Geometry: see drawing. Coordinates: mm, zero at the bounding-box minimum. A direction names the side the tool comes from. Coordinates: 2 decimals unless noted, no trailing zeros. Order: outer loops, then holes, each group sorted by start corner. A loop starts at its lowest first (then second) coordinate and runs counter-clockwise, first axis right, second up. Notation, with made-up numbers: (21, 51) -> (41, 51) arc R20 ccw to (41, 67) -> close; hole circle Ø10 at (75.25, -8). An arc over 180 degrees is marked (long way). Write each question's results on one line, items separated by ' | '.
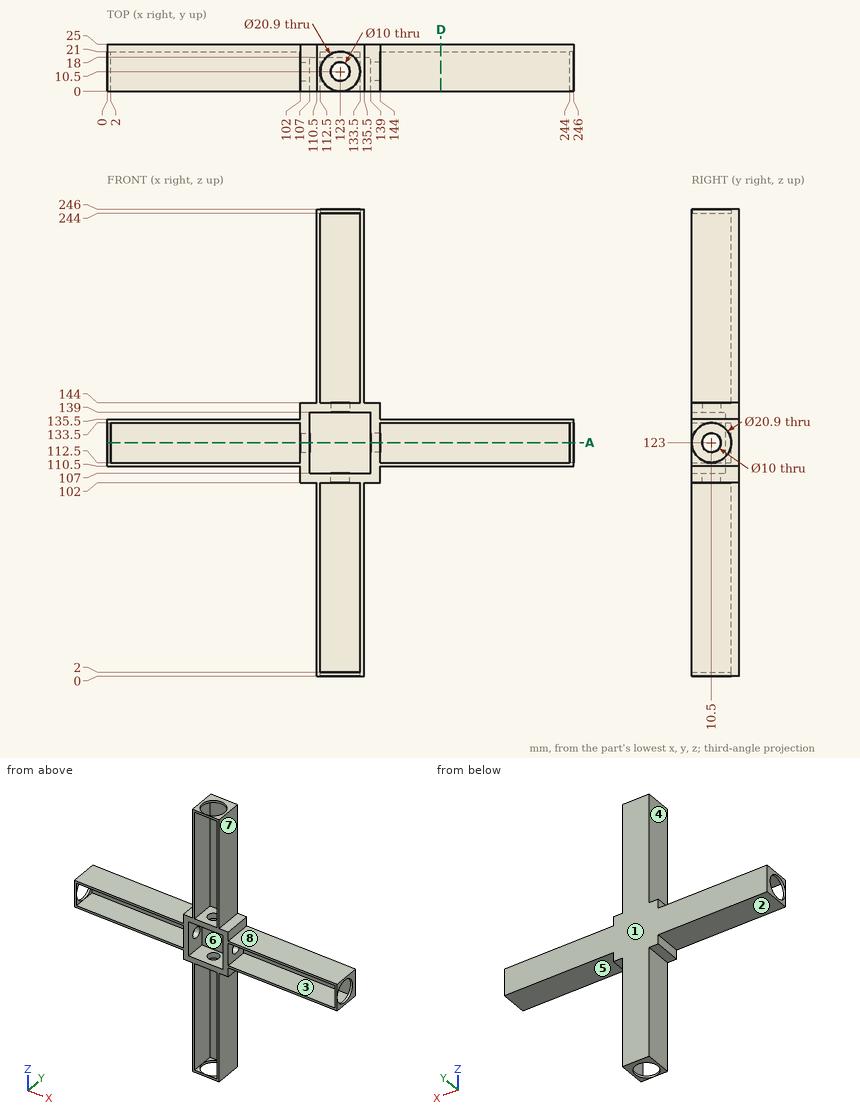
(1) Mould query, pull axis X, two halves, no side actions, for the marked faces 6, 7 and 8. Classes: +X half, -X half, draft (parallel to the pull), parting line (faces both ways), or undercut.
Return value:
face 6: undercut | face 7: +X half | face 8: draft
(2) Reachability of the marked faces 1, 2, 3, 4 and 5 from +Z, -Z, +X, -X, +Y, -Y: full face, straight path, thin tool, end or side. Return the list, or none.
Return value:
face 1: +Z, -Z, +X, -X, +Y | face 2: -Z, -X, +Y, -Y | face 3: -Y | face 4: +Z, -X, +Y, -Y | face 5: -Z, +X, +Y, -Y
(3) Cut plane D-D, the plane x = 176. Return loops of the section in (y, z).
Return value:
outline: (0, 110.5) -> (25, 110.5) -> (25, 135.5) -> (0, 135.5) -> (0, 133.5) -> (21, 133.5) -> (21, 112.5) -> (0, 112.5) -> close
(4) Line query: line 1 along Z through (x, y) = (73, 18); line 2 along X through (y, z) = (11.25, 116.5). Output: solid intervals per line, ascending. Write a range as from..to.
Return value:
line 1: 110.5..112.5, 133.5..135.5 | line 2: 102..107, 139..144
(5) Cut plane A-A, the plane z = 123. Count the separate pieces of the cut face and the enclosed holes in it, plus the area to 3 significant figures.
Return value:
separate pieces: 5 | enclosed holes: 0 | area: 1,190 mm2
(6) Pin query (flat end, axial travel): P1, Ø8, axis at x = 115, y = 22, coming from the -Z side; P2, Ø1.5, axis at x = 118, y = 9.5, coming from the +Z side; P3, Ø6.5, axis at x = 125.5, y = 13.5, coming from the -Z side; P4, Ø2, axis at y = 8, z = 77.5, coming from the +X side. Return the tip coordinate at first contact, or that it passes through.
Return value:
P1: z = 0 | P2: z = 144 | P3: z = 102 | P4: x = 135.5
